Here's how the part is built. I have some questions about the finished solid (model axes, mm). Round coordinates to 2 decimals unless told otherwise and drop trailing zeros. Order: outer loops, then holes, each group sorted by start corner. A loop starts at its lowest first (then second) coordinate and runs counter-clockwise, first axis right, second up. Notation, with made-up numbers: M 67,53 L 84,53 A18 cw 84,64 Z; hole C 63,21.25 d2. An arc over 180 degrees is marked long. Write item = value, one per line. Start each with the question number.
Item 1: I want a section at B-B, the plane x = 207. List the corners of the cut face in (y, z) for me, plus the area to 3 significant figures.
Item 2: I'm going to push flat-ended pins straight in: P1, Ø5, axis at x = 121.5, y = -218, coming from the -Z side; P2, Ø10, axis at x = 147.5, y = -239.5, coming from the +Z side. Where does each tip first touch, or does it pass through?
Item 3: Please list where these lines run through material, in increasing order: L1, parallel to Z at x = 215.5, y = -143; L2, parallel to X at y = -158.5, z = -44; L3, parallel to X at y = -177, z = 441.
Item 4: I want a section at C-C, the plane z = 427. List the corners of the cut face in (x, y) for me, plus the area to 3 significant figures.
Item 5: I want a section at A-A, the plane y = -207.5. List the corners of the cut face in (x, z) for me.
```python
from build123d import *

# Parameters (mm, degrees)
SKETCH1_W                = 229.923881951
SKETCH1_H                = 177.514761801
BOSS_EXTRUDE1_DEPTH      = 400
BOSS_EXTRUDE2_DEPTH      = 112
BOSS_EXTRUDE2_DEPTH_BACK = 503
SKETCH2_R                = 12.5


with BuildPart() as part:
    # Sketch1 → Boss-Extrude1 (new body)
    with BuildSketch(Plane.XY):
        with Locations((144.662099629, -170.086101065)):
            Rectangle(SKETCH1_W, SKETCH1_H)
    extrude(amount=BOSS_EXTRUDE1_DEPTH)

    # Sketch2 → Boss-Extrude2 (add, two sides: drawn at the far end of the back side and taken through both)
    with BuildSketch(Plane.XY.offset(400).offset(-BOSS_EXTRUDE2_DEPTH_BACK)):
        with Locations((144.662099628, -170.086101065)):
            Circle(SKETCH2_R)
    extrude(amount=BOSS_EXTRUDE2_DEPTH + BOSS_EXTRUDE2_DEPTH_BACK)


solid = part.part
```
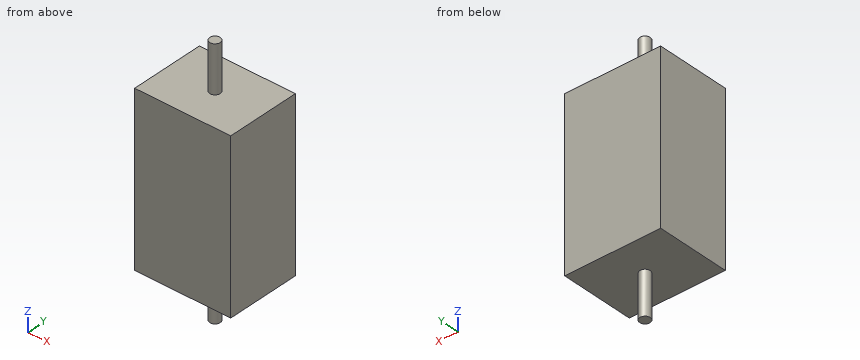
Filled in:
q1.outline = M -258.84,0 L -81.33,0 L -81.33,400 L -258.84,400 Z
q1.area = 71,000 mm^2
q2.P1 = 0
q2.P2 = 400
q3.L1 = 0 to 400
q3.L2 = 139.97 to 149.35
q3.L3 = 134.25 to 155.08
q4.outline = C 144.66,-170.09 d25
q4.area = 491 mm^2
q5.outline = M 29.7,0 L 259.62,0 L 259.62,400 L 29.7,400 Z
